Study the drawing (mm; zero at the part's minimum x, y, z) and answer. A direction names the side the tool comes from. Round coordinates to 2 decimals unless told otherwise and drop trailing zeros. Write each loop counter-clockwise with the first axis right and the second up, starting at its lowest first coordinate (ties: lowest second). Pieces come first, ordered by that corner, then holes.
(1) A cutting plane is placed at B-B, the plane x = 36.5. Give the vertices of the cut face in (y, z).
(2) A cutting plane is placed at C-C, the plane y = 33.5. Give the vertices of the cut face in (x, z).
(3) A cutting plane is placed at A-A, the plane z = 12. Give the vertices of the cut face in (x, y), and give its area (3 significant figures).
(4) Find the intervals of material crossed by probe 1 along X at (y, z) = (32.9, 12); probe 2 along Z at (x, y) = (36.5, 32.6); probe 3 along Y at (x, z) = (25, 3), in increasing order.
(5) Each of these flat-tipped pins is pushed along its axis until it touches: pin 1 Ø9.5 at (x, y) = (20, 16.5) entering from -Z; pin 2 Ø12 at (x, z) = (8.5, 22.5) entering from -Y. Where does it stop, or does it pass through?
(6) For the marked faces 1 and 2, determine the directions among +Z, -Z, +X, -X, +Y, -Y from which every point of the face is accessible in a straight line to the end or side of a thin tool.
(7) A cutting plane is placed at D-D, the plane x = 24. Give the vertices of the cut face in (y, z).
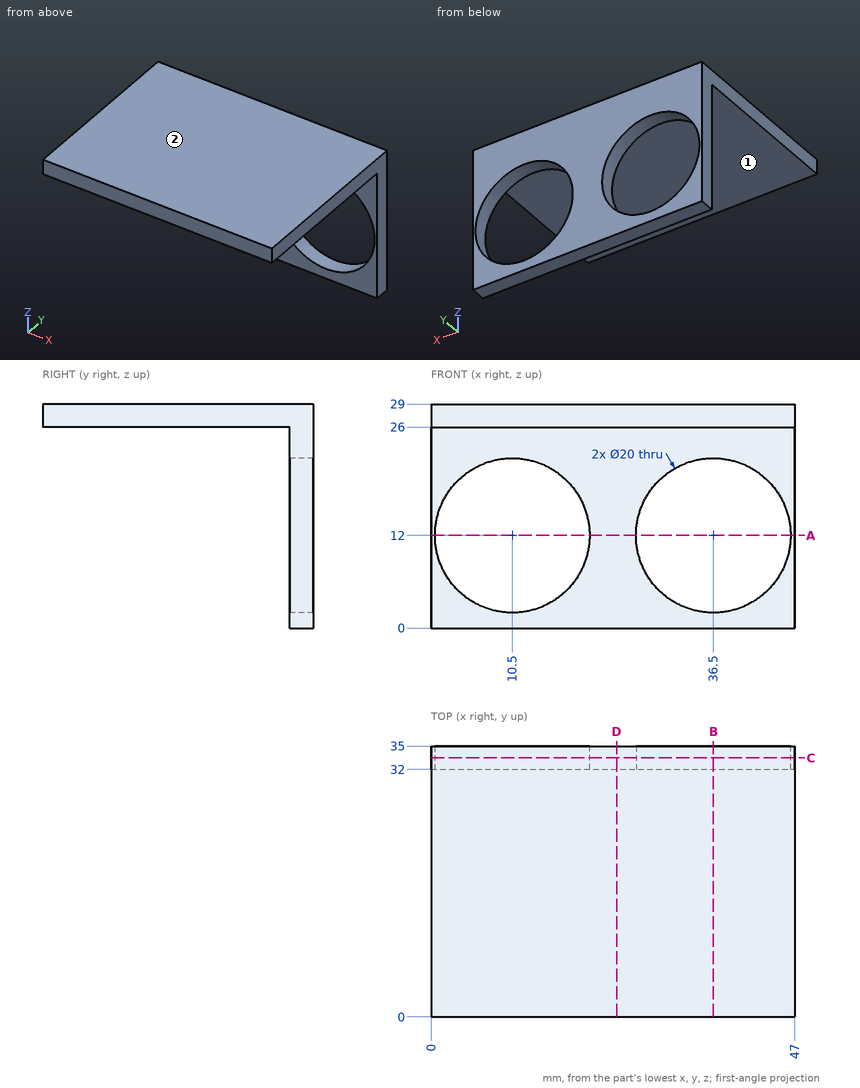
Solutions:
1. outline: (0, 26) - (32, 26) - (32, 22) - (35, 22) - (35, 29) - (0, 29) - close; (32, 0) - (35, 0) - (35, 2) - (32, 2) - close
2. outline: (0, 0) - (47, 0) - (47, 29) - (0, 29) - close; hole circle Ø20 at (10.5, 12); hole circle Ø20 at (36.5, 12)
3. outline: (0, 32) - (0.5, 32) - (0.5, 35) - (0, 35) - close; (20.5, 32) - (26.5, 32) - (26.5, 35) - (20.5, 35) - close; (46.5, 32) - (47, 32) - (47, 35) - (46.5, 35) - close
3. area: 21.0 mm2
4. probe 1: x = 0 to 0.5, 20.5 to 26.5, 46.5 to 47
4. probe 2: z = 0 to 2, 22 to 29
4. probe 3: y = 32 to 35
5. pin 1: stops at z = 26
5. pin 2: stops at y = 0
6. face 1: -Z, +X, -X, -Y
6. face 2: +Z, +X, -X, +Y, -Y
7. outline: (0, 26) - (32, 26) - (32, 0) - (35, 0) - (35, 29) - (0, 29) - close
